from build123d import *

# Parameters (mm, degrees)
FILLET1_R               = 2.54
CUT_EXTRUDE1_REACH      = 170.913
CUT_EXTRUDE1_END_RADIUS = 43.0260506
SKETCH2_R               = 1.5875
CUT_EXTRUDE2_REACH      = 170.913
CUT_EXTRUDE2_END_RADIUS = 43.0260506
SKETCH3_R               = 5.207


with BuildPart() as part:
    # Model → Revolve1 (revolve)
    with BuildSketch(Plane.XY, mode=Mode.PRIVATE) as revolve1_sk:
        with BuildLine():
            Line((-112.522, 43.0260506), (-73.383883216, 43.0260506))
            ThreePointArc((-73.383883216, 43.0260506), (-52.084113896, 40.221883155), (-32.235888265, 32.000480144))
            Line((-32.235888265, 32.000480144), (-13.143390216, 20.97742306))
            ThreePointArc((-13.143390216, 20.97742306), (-6.833614784, 18.363828893), (-0.062391821, 17.4723806))
            Line((-0.062391821, 17.4723806), (-0.049911, 17.4723806))
            ThreePointArc((-0.049911, 17.4723806), (1.272148929, 17.604626372), (2.541818849, 17.996123109))
            add(Edge.make_bspline(
                [(2.541818849, 17.996123109), (36.7084102, 32.3929756), (72.4744296, 40.360473)],
                knots=[0, 0, 0, 1, 1, 1], degree=2))
            Line((72.4744296, 40.360473), (69.712974983, 52.756616287))
            add(Edge.make_bspline(
                [(-1.156547602, 30.216919323), (4.596059921, 32.619985433), (16.22720374, 37.184585521), (39.705039846, 45.226383183), (57.634347708, 50.065893836), (69.712974983, 52.756616287)],
                knots=[0.017508698, 0.017508698, 0.017508698, 0.017508698, 0.263131524, 0.508754349, 1, 1, 1, 1], degree=3))
            ThreePointArc((-1.156547602, 30.216919323), (-4.072604577, 30.78355815), (-6.793390995, 31.975946137))
            Line((-6.793390995, 31.975946137), (-25.885889044, 42.999003222))
            Line((-25.885889044, 42.999003222), (-48.255103535, 55.7260506))
            Line((-48.255103535, 55.7260506), (-112.522, 55.7260506))
            Line((-112.522, 55.7260506), (-112.522, 43.0260506))
        make_face()
    revolve(revolve1_sk.sketch.rotate(Axis((-112.522, 0, 0), (1, 0, 0)), 90), axis=Axis((-112.522, 0, 0), (1, 0, 0)))

    # Fillet1
    fillet1_edges = [part.edges().sort_by_distance(p)[0] for p in [
        (-112.522, 0, -55.7260506),
    ]]
    fillet(fillet1_edges, radius=FILLET1_R)

    # Cut-Extrude1: up to this cylinder (the profile starts outside it)
    cut_extrude1_end = Plane(origin=(-102.997, 0, 0), z_dir=(-1, 0, 0)) * Cylinder(CUT_EXTRUDE1_END_RADIUS, 428.8781012, mode=Mode.PRIVATE)
    # Sketch2 → Cut-Extrude1 (cut, up to the surface)
    with BuildSketch(Plane(origin=(0, -3.172071011, 55.635696104), x_dir=(-1, 0, 0), z_dir=(0, -0.056922587846044495, 0.9983785950193993)), mode=Mode.PRIVATE) as cut_extrude1_sk1:
        with Locations(Location((102.997, 0, 0), (0, 0, 90))):
            Circle(SKETCH2_R)
    cut_extrude1_tool1 = extrude(cut_extrude1_sk1.sketch, amount=-CUT_EXTRUDE1_REACH, mode=Mode.PRIVATE) - cut_extrude1_end
    add(cut_extrude1_tool1.solids().sort_by_distance((-102.997, -3.172071, 55.635696))[0], mode=Mode.SUBTRACT)

    # Cut-Extrude2: up to this cylinder (the profile starts outside it)
    cut_extrude2_end = Plane(origin=(-106.172, 0, 0), z_dir=(-1, 0, 0)) * Cylinder(CUT_EXTRUDE2_END_RADIUS, 428.8781012, mode=Mode.PRIVATE)
    # Sketch3 → Cut-Extrude2 (cut, up to the surface)
    with BuildSketch(Plane(origin=(0, -55.635696104, -3.172071011), x_dir=(-1, 0, 0), z_dir=(0, -0.9983785950193991, -0.05692258784604798)), mode=Mode.PRIVATE) as cut_extrude2_sk1:
        with Locations(Location((106.172, 0, 0), (0, 0, 90))):
            Circle(SKETCH3_R)
    cut_extrude2_tool1 = extrude(cut_extrude2_sk1.sketch, amount=-CUT_EXTRUDE2_REACH, mode=Mode.PRIVATE) - cut_extrude2_end
    add(cut_extrude2_tool1.solids().sort_by_distance((-106.172, -55.635696, -3.172071))[0], mode=Mode.SUBTRACT)


solid = part.part
Input: part model. Units: mm. Frame: model coordinates. A direction names the side the tool comes from. Round coordinates to 2 decimals unless told otherwise and drop trailing zeros. Order: outer loops, then holes, each group sorted by start corner. A loop starts at its lowest first (then second) coordinate and runs counter-clockwise, first axis right, second up. Notation, with made-up numbers: (28, -36) - (56, -36) arc R11 cw to (56, -32) - close; hole circle Ø7 at (37.5, 70.5). An arc over 180 degrees is marked (long way). Use a Markdown table: item, result.
1. Section A-A on x = -21. Return the cut outline in (y, z).
Evaluation:
| item | result |
|---|---|
| outline | circle Ø80.36 at (0, 0); hole circle Ø51.03 at (0, 0) |
2. Mould query, pull axis Y, two halves, no side actions, for faces 4 (the face through (-27.285, 38.854, 20.209)), 5 (the face through (-110.79, -49.09, -5.21)), 6 (the face through (-112.522, 43, -4)). Classes: +Y half, -Y half, draft (parallel to the pull), parting line (faces both ways), or undercut.
Evaluation:
| item | result |
|---|---|
| face 4 | parting line |
| face 5 | undercut |
| face 6 | draft |
3. Material intervals for probe 1 along Z at (x, y) = (-31, 20.5); probe 2 along Y at (x, z) = (44.5, -20); probe 3 along Y at (x, z) = (-0.05, 0), sorted ascending.
Evaluation:
| item | result |
|---|---|
| probe 1 | -41.08 to -23.64, 23.64 to 41.08 |
| probe 2 | -41.77 to -26.34, 26.34 to 41.77 |
| probe 3 | -30.68 to -17.47, 17.47 to 30.68 |
4. First-contact query: pin 1 (1 mm diameter, centred on x = 49.5, z = 4, fed in from +Y); pin 2 (2 mm diameter, centred on x = -66, z = -27.5, fed in from -Y); pin 3 (1.5 mm diameter, centred on x = 9.5, y = 19.5, fed in from -Z); pin 4 (8 mm diameter, centred on y = -2, z = 13, fed in from -X). Flat tips, straight axial feed; report the tip coordinate or a pass-through.
Evaluation:
| item | result |
|---|---|
| pin 1 | y = 47.7 |
| pin 2 | y = -49.02 |
| pin 3 | z = -29.07 |
| pin 4 | through |
5. Access query for faces 1 (the face through (-92.679, 38.172, 19.854)), 2 (the face through (-7.99, -9.81, 31.16)), 3 (the face through (-79.55, 49.44, 25.71)). Directions: +Z, -Z, +X, -X, +Y, -Y. A direction counts if a zero-diameter tool reaches every point of the face in a straight line with its end or side. Return the directions, or none.
Evaluation:
| item | result |
|---|---|
| face 1 | -X |
| face 2 | none |
| face 3 | +X, -X |
